Verification items for this drawing (mm, ordinates from the low corner). A direction names the side the tool comes from. Give positions to 0.01 mm unless a question says otherwise; leave off trailing zeros. Loops run counter-clockwise (first coordinate to the right, second up) from the corner with the lowest first, then second, coordinate; pieces in that order, holes last. Notation, with made-up numbers: M 64,-12.75 L 95,-12.75 A35 cw 95,25.25 Z; hole C 54,57.25 d5. An arc over 180 degrees is marked long. Use one line per item in the form item = value.
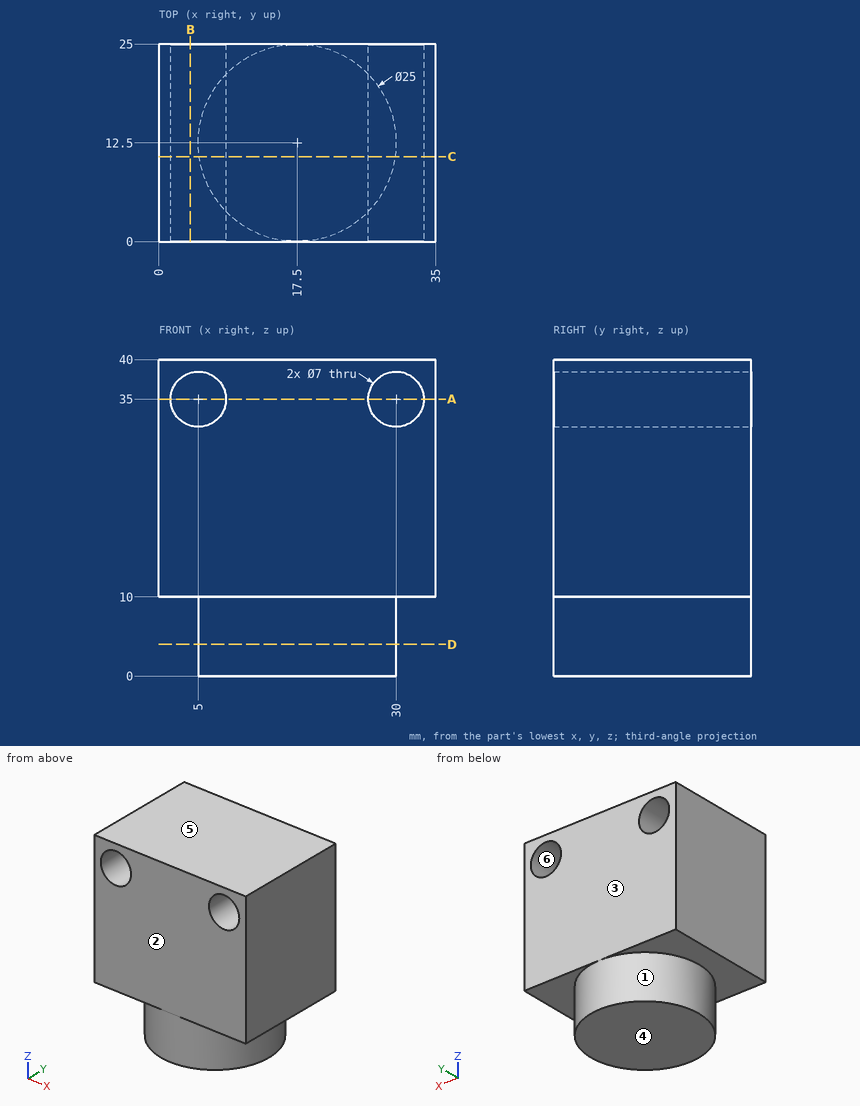
1) Section check C-C (y = 10.75). Record the cut outline in (x, z).
Evaluation:
outline = M 0,10 L 5.12,10 L 5.12,0 L 29.88,0 L 29.88,10 L 35,10 L 35,40 L 0,40 Z; hole C 5,35 d7; hole C 30,35 d7
2) Section check D-D (z = 4). Record the cut outline in (x, y), then the cut area to 3 significant figures.
Evaluation:
outline = C 17.5,12.5 d25
area = 491 mm^2
3) Scan lines: line 1 (X direction, y = 11.5, z = 35); line 2 (Z direction, x = 30, y = 10.75); line 3 (Z direction, x = 3, y = 19). Record each from-to range of solid material in increasing order.
Evaluation:
line_1 = 0 to 1.5, 8.5 to 26.5, 33.5 to 35
line_2 = 10 to 31.5, 38.5 to 40
line_3 = 10 to 32.13, 37.87 to 40
4) Release check for a two-part mould opening along Z. For the marked faces 3, 4, 5 and 6 record: pulls with the +Z half, pulls with the -Z half, needs draft (parallel to the pull), parting line crosses it, or undercut.
Evaluation:
face_3 = needs draft
face_4 = pulls with the -Z half
face_5 = pulls with the +Z half
face_6 = undercut
5) Section check A-A (z = 35). Record the cut outline in (x, y).
Evaluation:
outline = M 0,0 L 1.5,0 L 1.5,25 L 0,25 Z; M 8.5,0 L 26.5,0 L 26.5,25 L 8.5,25 Z; M 33.5,0 L 35,0 L 35,25 L 33.5,25 Z
6) Section check B-B (x = 4). Record the cut outline in (y, z).
Evaluation:
outline = M 0,10 L 25,10 L 25,31.65 L 0,31.65 Z; M 0,38.35 L 25,38.35 L 25,40 L 0,40 Z
7) Set-up check for the marked faces 1 and 2: record each of +Z, -Z, +X, -X, +Y, -Y from which the full face is reachable in a straight line by a thin tool's end or side.
Evaluation:
face_1 = -Z
face_2 = +Z, -Z, +X, -X, -Y
